Verification items for this drawing (mm, ordinates from the low corner). A direction names the side the tool comes from. Round coordinates to 2 decimals unless told otherwise and drop trailing zeros. Order: outer loops, then holes, each group sorted by start corner. A loop starts at its lowest first (then second) coordinate and runs counter-clockwise, first axis right, second up. Notation, with made-up numbers: (48, -3) -> (93, -3) arc R26 cw to (93, 29) -> close; hole circle Ø3 at (-2.75, 20). An arc over 180 degrees is marked (long way). Use a Markdown table: item, result. Add a question column.
Item 1: Sectioned sample at D-D, the plane y = 3. State how many separate pieces and enclosed holes the cut face has, and give its area (3 significant figures).
Item 2: Gauge pin test, flat ends, axial feed: pin 1 Ø4 at (x, z) = (9.19, 51.87) entering from -Y; pin 2 Ø3.5 at (y, z) = (20.5, 51) entering from -X; pin 3 Ø6 at (y, z) = (21, 36) entering from -X. Record the tip position at first contact, or that the pin passes through.
Item 3: Material ranges on probe 1 along X at (y, z) = (16, 36.25); probe 2 along Z at (x, y) = (36, 19); probe 3 along Z at (x, y) = (48.5, 5.5) (1 decimal), recorded low to high. Write a range as [from, to].
Item 4: Sectioned sample at C-C, the plane y = 8. Record the cut outline in (x, z), and give its area (3 significant figures).
Item 5: Sectioned sample at B-B, the plane x = 36.25. Record the cut outline in (y, z).
Item 6: Sectioned sample at A-A, the plane z = 36.25. Record the cut outline in (x, y).
Item 7: Set-up check for the marked faces 1 and 2: record each of +Z, -Z, +X, -X, +Y, -Y from which the full face is reachable in a straight line by a thin tool's end or side.
Item 8: Mould release check, pull along X, two halves, no side actions. Record for the marked faces 3, 4, 5 and 6: pulls with the +X half, pulls with the -X half, needs draft (parallel to the pull), parting line crosses it, or undercut.
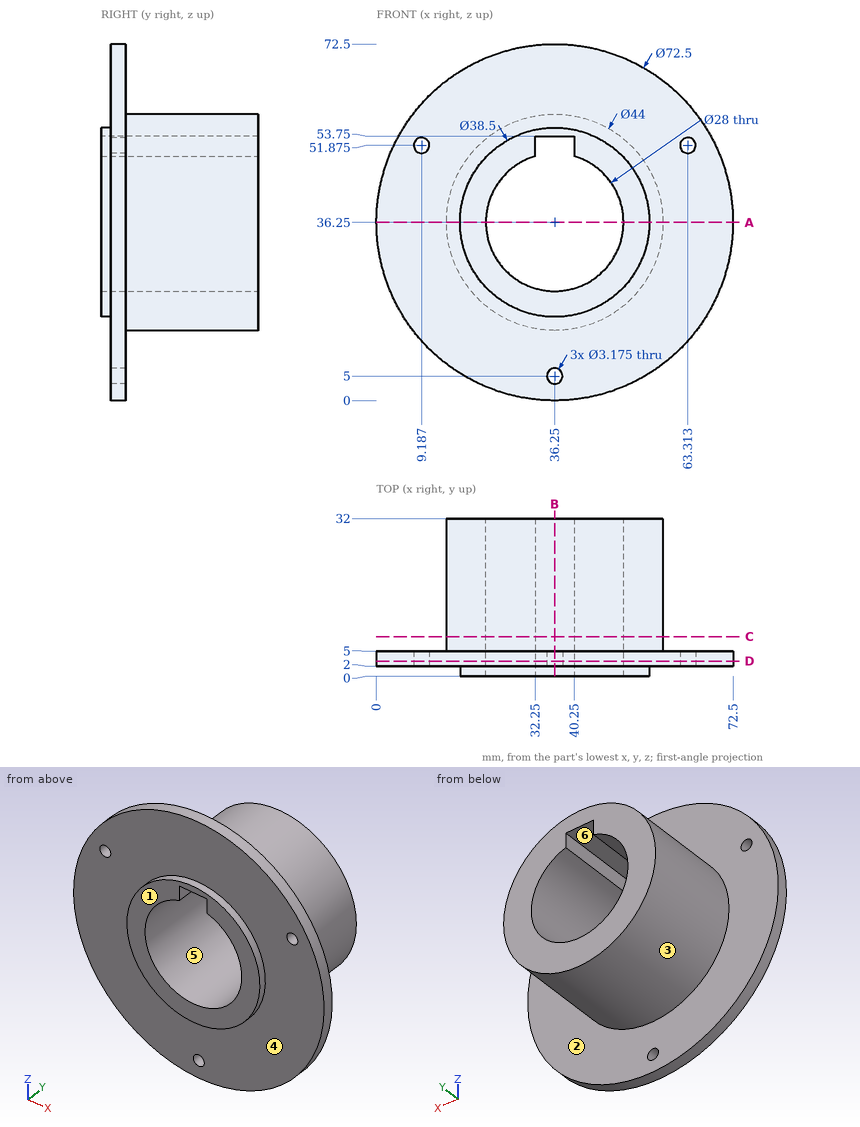
Found:
| question | item | result |
|---|---|---|
| 1 | separate pieces | 1 |
| 1 | enclosed holes | 4 |
| 1 | area | 3,460 mm2 |
| 2 | pin 1 | stops at y = 2 |
| 2 | pin 2 | stops at x = 18.5 |
| 2 | pin 3 | stops at x = 14.25 |
| 3 | probe 1 | x = [14.25, 22.25], [50.25, 58.25] |
| 3 | probe 2 | z = [14.25, 22.25], [53.75, 58.25] |
| 3 | probe 3 | z = [18, 29.5], [43, 54.5] |
| 4 | outline | circle Ø44 at (36.25, 36.25); hole (32.25, 49.67) arc R14 ccw (long way) to (40.25, 49.67) -> (40.25, 53.75) -> (32.25, 53.75) -> close |
| 4 | area | 875 mm2 |
| 5 | outline | (0, 17) -> (2, 17) -> (2, 6.59) -> (5, 6.59) -> (5, 14.25) -> (32, 14.25) -> (32, 22.25) -> (0, 22.25) -> close; (0, 53.75) -> (32, 53.75) -> (32, 58.25) -> (5, 58.25) -> (5, 72.5) -> (2, 72.5) -> (2, 55.5) -> (0, 55.5) -> close; (2, 0) -> (5, 0) -> (5, 3.41) -> (2, 3.41) -> close |
| 6 | outline | (0, 2) -> (17, 2) -> (17, 0) -> (22.25, 0) -> (22.25, 32) -> (14.25, 32) -> (14.25, 5) -> (0, 5) -> close; (50.25, 0) -> (55.5, 0) -> (55.5, 2) -> (72.5, 2) -> (72.5, 5) -> (58.25, 5) -> (58.25, 32) -> (50.25, 32) -> close |
| 7 | face 1 | +Z, -Z, +X, -X, -Y |
| 7 | face 2 | +Y |
| 8 | face 3 | parting line crosses it |
| 8 | face 4 | needs draft |
| 8 | face 5 | undercut |
| 8 | face 6 | undercut |
